The model under review builds one solid part; all positions refer to its coordinate system, in mm. Face numbers are marked on the shaded views. A direction names the side the tool comes from. Give positions to 0.01 mm unless a question says otherwise; leave off trailing zeros. Write each loop counter-clockwise with the first axis right and the second up, starting at its lowest first coordinate (ties: lowest second). Pieces come first, ordered by that corner, then holes. Notation, with made-up numbers: (16.5, 21.5) - (32.5, 21.5) arc R11 ccw to (32.5, 37.5) - close; hole circle Ø7 at (77.25, -19.75). An arc over 180 degrees is marked (long way). Write item = value, one per line.
```python
from build123d import *

# Parameters (mm, degrees)
SM_BASE_FLANGE_1_DEPTH      = 40
CUT_EXTRUDE_3_DEPTH         = 10
CUT_EXTRUDE_1_DEPTH         = 76.219678276
SKETCH_7_R                  = 1.6
CUT_EXTRUDE_2_DEPTH         = 76.219678276
SKETCH_9_R                  = 1.6
CUT_EXTRUDE_4_DEPTH         = 76.219678276
PATTERN_LINEAR_1_COUNT      = 2
PATTERN_LINEAR_1_PITCH      = 30
PATTERN_LINEAR_1_COUNT_DIR2 = 2
PATTERN_LINEAR_1_PITCH_DIR2 = 24
FILLET_1_R                  = 5


# Sheet-metal steps are written as plain solids
with BuildPart() as part:
    # Sketch 1 → 基材-凸緣1 (new body)
    with BuildSketch(Plane.XY):
        with BuildLine():
            Line((43, 0), (4, 0))
            ThreePointArc((4, 0), (1.171572875, 1.171572875), (0, 4))
            Line((0, 4), (0, 47))
            Line((0, 47), (3, 47))
            Line((3, 47), (3, 4))
            ThreePointArc((3, 4), (3.292893219, 3.292893219), (4, 3))
            Line((4, 3), (43, 3))
            Line((43, 3), (43, 0))
        make_face()
    extrude(amount=SM_BASE_FLANGE_1_DEPTH)

    # 草圖8 → 除料-伸長3 (cut)
    with BuildSketch(Plane.ZY):
        with BuildLine():
            Line((0, 47), (0, 27))
            ThreePointArc((0, 27), (5.857864376, 41.142135624), (20, 47))
            Line((20, 47), (0, 47))
        make_face()
        with BuildLine():
            ThreePointArc((20, 47), (34.142135624, 41.142135624), (40, 27))
            Line((40, 27), (40, 47))
            Line((40, 47), (20, 47))
        make_face()
    extrude(amount=-CUT_EXTRUDE_3_DEPTH, mode=Mode.SUBTRACT)

    # 草圖6 → 除料-伸長1 (cut, through all)
    with BuildSketch(Plane.ZY):
        with BuildLine():
            Line((26.5, 32.5), (26.5, 18.5))
            ThreePointArc((26.5, 18.5), (20, 12), (13.5, 18.5))
            Line((13.5, 18.5), (13.5, 32.5))
            ThreePointArc((13.5, 32.5), (20, 39), (26.5, 32.5))
        make_face()
    extrude(amount=-CUT_EXTRUDE_1_DEPTH, mode=Mode.SUBTRACT)

    # 草圖7 → 除料-伸長2 (cut, through all)
    with BuildSketch(Plane.ZY):
        with Locations((4.5, 25.5)):
            Circle(SKETCH_7_R)
        with Locations((12.25, 12.076606241)):
            Circle(SKETCH_7_R)
        with Locations((27.75, 12.076606241)):
            Circle(SKETCH_7_R)
        with Locations((35.5, 25.5)):
            Circle(SKETCH_7_R)
        with Locations((27.75, 38.923393759)):
            Circle(SKETCH_7_R)
        with Locations((12.25, 38.923393759)):
            Circle(SKETCH_7_R)
    extrude(amount=-CUT_EXTRUDE_2_DEPTH, mode=Mode.SUBTRACT)

    # 草圖9 → 除料-伸長4 (cut, through all)
    with BuildSketch(Plane.XZ):
        with Locations(Location((32, 35, 0), (0, 0, 270))):
            Circle(SKETCH_9_R)
    cut_extrude_4 = extrude(amount=-CUT_EXTRUDE_4_DEPTH, mode=Mode.SUBTRACT)

    # 直線複製排列1: Cut-Extrude 4 2 × 2
    with Locations(*[(-j * PATTERN_LINEAR_1_PITCH_DIR2, 0, -i * PATTERN_LINEAR_1_PITCH) for i in range(PATTERN_LINEAR_1_COUNT) for j in range(PATTERN_LINEAR_1_COUNT_DIR2) if (i, j) != (0, 0)]):
        add(cut_extrude_4, mode=Mode.SUBTRACT)

    # 圓角1
    fillet_1_edges = [part.edges().sort_by_distance(p)[0] for p in [
        (43, 1.5, 40),
        (43, 1.5, 0),
    ]]
    fillet(fillet_1_edges, radius=FILLET_1_R)


solid = part.part
```
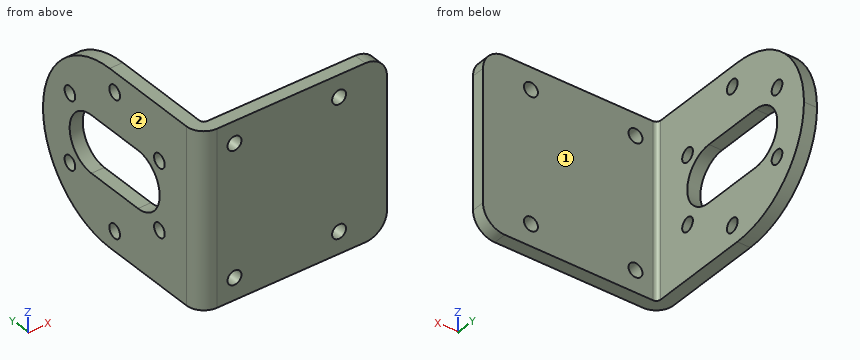
1. Take a section at C-C on z = 21. Give the boundary of the cut face in (x, y), and give its area (3 significant figures).
Findings below:
outline = (0, 4) arc R4 ccw to (4, 0) - (43, 0) - (43, 3) - (4, 3) arc R1 cw to (3, 4) - (3, 12.08) - (0, 12.08) - close; (0, 38.92) - (3, 38.92) - (3, 46.97) - (0, 46.97) - close
area = 177 mm²
2. For line 1 (Y direction, x = 1.4, z = 27.75); line 2 (Y direction, x = 2.2, z = 27.75); line 3 (Y direction, x = 18.5, z = 31), list the stretches that pass through material, from the lowest coordinate up. Write a range as from..to.
Findings below:
line_1 = 0.96..10.48, 13.68..37.32, 40.52..45.44
line_2 = 0.43..10.48, 13.68..37.32, 40.52..45.44
line_3 = 0..3
3. Take a section at B-B on z = 12.25. Give the boundary of the cut face in (x, y).
Findings below:
outline = (0, 4) arc R4 ccw to (4, 0) - (43, 0) - (43, 3) - (4, 3) arc R1 cw to (3, 4) - (3, 10.48) - (0, 10.48) - close; (0, 13.68) - (3, 13.68) - (3, 37.32) - (0, 37.32) - close; (0, 40.52) - (3, 40.52) - (3, 45.44) - (0, 45.44) - close
4. Machinability: for the marked faces 1 and 2, which of the approach directions +Z, -Z, +X, -X, +Y, -Y give a long, thin tool a straight path to every point of the face, cutting with its end or side? Answer none if there is none.
Findings below:
face_1 = +Z, -Z, +X, +Y
face_2 = +Z, -Z, -X, +Y, -Y
5. Take a section at A-A on y = 21. Give the boundary of the cut face in (x, z), and give its area (3 significant figures).
Findings below:
outline = (0, 0) - (3, 0) - (3, 13.5) - (0, 13.5) - close; (0, 26.5) - (3, 26.5) - (3, 40) - (0, 40) - close
area = 81.0 mm²
6. Insertion check: P1, Ø3, axis at y = 25.5, z = 35.5, coming from the -X side; P2, Ø3, axis at y = 35.5, z = 33, coming from the +X side; P3, Ø3, axis at y = 13.5, z = 24, coming from the -X side; P4, Ø8, axis at x = 28, z = 9.5, coming from the +Y side. Each pin has a flat end and moves straight along its axis. Give the tip position at first contact, or say it passes through.
Findings below:
P1 = through
P2 = 3
P3 = 0
P4 = 3
7. Take a section at D-D on x = 16. Give the boundary of the cut face in (y, z).
Findings below:
outline = (0, 0) - (3, 0) - (3, 40) - (0, 40) - close
